Geometry check sheet. Reference: the model listing, model coordinates, mm. Give positions to 0.01 mm unless a question says otherwise; leave off trailing zeros. Write each loop counter-clockwise with the first axis right and the second up, starting at its lowest first coordinate (ties: lowest second). Pieces come first, ordered by that corner, then holes. Notation, with made-up numbers: M -14.5,28 L 3.5,28 A4 ccw 3.5,32 Z; hole C 89.5,51.25 d4. An arc over 180 degrees is marked long. Write each question's results on one line, items separated by ' | '.
```python
from build123d import *

# Parameters (mm, degrees)
SKETCH1_W            = 155
SKETCH1_H            = 103
SKETCH1_W_2          = 147
SKETCH1_H_2          = 95
BOSS_EXTRUDE2_DEPTH  = 3
SKETCH3_W            = 13
SKETCH3_H            = 3
BOSS_EXTRUDE5_DEPTH  = 22.5
SKETCH4_W            = 12
SKETCH4_H            = 3
BOSS_EXTRUDE6_DEPTH  = 22.5
SKETCH5_W            = 20
SKETCH5_H            = 32
SKETCH5_R            = 2.5
BOSS_EXTRUDE7_DEPTH  = 3
SKETCH6_W            = 20
SKETCH6_H            = 33
SKETCH6_R            = 2.5
BOSS_EXTRUDE8_DEPTH  = 3
SKETCH2_3_R          = 7
SKETCH2_3_R_2        = 1.25
BOSS_EXTRUDE11_DEPTH = 3
SKETCH2_R            = 7
SKETCH2_R_2          = 1.25
BOSS_EXTRUDE10_DEPTH = 3


with BuildPart() as part:
    # Sketch1 → Boss-Extrude2 (new body)
    with BuildSketch(Plane(origin=(0, 0, 0), x_dir=(1, 0, 0), z_dir=(0, 1, 0))):
        with Locations((77.5, 51.5)):
            Rectangle(SKETCH1_W, SKETCH1_H)
        with Locations((77.5, 51.5)):
            Rectangle(SKETCH1_W_2, SKETCH1_H_2, mode=Mode.SUBTRACT)
    extrude(amount=BOSS_EXTRUDE2_DEPTH)

    # Sketch3 → Boss-Extrude5 (add)
    with BuildSketch(Plane.ZY):
        with Locations((-51, 1.5)):
            Rectangle(SKETCH3_W, SKETCH3_H)
    extrude(amount=BOSS_EXTRUDE5_DEPTH)

    # Sketch4 → Boss-Extrude6 (add)
    with BuildSketch(Plane(origin=(155, 0, 0), x_dir=(0, 0, -1), z_dir=(1, 0, 0))):
        with Locations((51.5, 1.5)):
            Rectangle(SKETCH4_W, SKETCH4_H)
    extrude(amount=BOSS_EXTRUDE6_DEPTH)

    # Sketch5 → Boss-Extrude7 (add)
    with BuildSketch(Plane(origin=(0, 3, 0), x_dir=(1, 0, 0), z_dir=(0, 1, 0))):
        with Locations((187.5, 51.5)):
            Rectangle(SKETCH5_W, SKETCH5_H)
        with Locations(Location((187.5, 60.5, 0), (0, 0, 270))):
            Circle(SKETCH5_R, mode=Mode.SUBTRACT)
        with Locations(Location((187.5, 42.5, 0), (0, 0, 270))):
            Circle(SKETCH5_R, mode=Mode.SUBTRACT)
    extrude(amount=-BOSS_EXTRUDE7_DEPTH)

    # Sketch6 → Boss-Extrude8 (add)
    with BuildSketch(Plane(origin=(0, 3, 0), x_dir=(1, 0, 0), z_dir=(0, 1, 0))):
        with Locations((-32.378431073, 51.050390221)):
            Rectangle(SKETCH6_W, SKETCH6_H)
        with Locations(Location((-32.5, 60.5, 0), (0, 0, 270))):
            Circle(SKETCH6_R, mode=Mode.SUBTRACT)
        with Locations(Location((-32.5, 42.5, 0), (0, 0, 270))):
            Circle(SKETCH6_R, mode=Mode.SUBTRACT)
    extrude(amount=-BOSS_EXTRUDE8_DEPTH)

    # Sketch2_3 → Boss-Extrude11 (add)
    # profile 1 of 4: a face of its own
    with BuildSketch(Plane(origin=(0, 3, 0), x_dir=(1, 0, 0), z_dir=(0, 1, 0))):
        with Locations((8, 8)):
            Circle(SKETCH2_3_R)
        with Locations(Location((8, 8, 0), (0, 0, 270))):
            Circle(SKETCH2_3_R_2, mode=Mode.SUBTRACT)
    # profile 2 of 4: a face of its own
    with BuildSketch(Plane(origin=(0, 3, 0), x_dir=(1, 0, 0), z_dir=(0, 1, 0))):
        with Locations((146, 8.25)):
            Circle(SKETCH2_3_R)
        with Locations(Location((146, 8.25, 0), (0, 0, 270))):
            Circle(SKETCH2_3_R_2, mode=Mode.SUBTRACT)
    # profile 3 of 4: a face of its own
    with BuildSketch(Plane(origin=(0, 3, 0), x_dir=(1, 0, 0), z_dir=(0, 1, 0))):
        with Locations((8, 94.75)):
            Circle(SKETCH2_3_R)
        with Locations(Location((8, 94.75, 0), (0, 0, 270))):
            Circle(SKETCH2_3_R_2, mode=Mode.SUBTRACT)
    # profile 4 of 4: a face of its own
    with BuildSketch(Plane(origin=(0, 3, 0), x_dir=(1, 0, 0), z_dir=(0, 1, 0))):
        with Locations((146, 94.75)):
            Circle(SKETCH2_3_R)
        with Locations(Location((146, 94.75, 0), (0, 0, 270))):
            Circle(SKETCH2_3_R_2, mode=Mode.SUBTRACT)
    extrude(amount=-BOSS_EXTRUDE11_DEPTH)

    # Sketch2 → Boss-Extrude10 (add)
    # profile 1 of 4: a face of its own
    with BuildSketch(Plane(origin=(0, 3, 0), x_dir=(1, 0, 0), z_dir=(0, 1, 0))):
        with Locations((8, 8)):
            Circle(SKETCH2_R)
        with Locations(Location((8, 8, 0), (0, 0, 270))):
            Circle(SKETCH2_R_2, mode=Mode.SUBTRACT)
    # profile 2 of 4: a face of its own
    with BuildSketch(Plane(origin=(0, 3, 0), x_dir=(1, 0, 0), z_dir=(0, 1, 0))):
        with Locations((146, 8.25)):
            Circle(SKETCH2_R)
        with Locations(Location((146, 8.25, 0), (0, 0, 270))):
            Circle(SKETCH2_R_2, mode=Mode.SUBTRACT)
    # profile 3 of 4: a face of its own
    with BuildSketch(Plane(origin=(0, 3, 0), x_dir=(1, 0, 0), z_dir=(0, 1, 0))):
        with Locations((8, 94.75)):
            Circle(SKETCH2_R)
        with Locations(Location((8, 94.75, 0), (0, 0, 270))):
            Circle(SKETCH2_R_2, mode=Mode.SUBTRACT)
    # profile 4 of 4: a face of its own
    with BuildSketch(Plane(origin=(0, 3, 0), x_dir=(1, 0, 0), z_dir=(0, 1, 0))):
        with Locations((146, 94.75)):
            Circle(SKETCH2_R)
        with Locations(Location((146, 94.75, 0), (0, 0, 270))):
            Circle(SKETCH2_R_2, mode=Mode.SUBTRACT)
    extrude(amount=-BOSS_EXTRUDE10_DEPTH)


solid = part.part
```
Q1. Release check for a two-part mould opening along X. For faces 1 (the face through (13, 1.5, -12.9)), 2 (the face through (77, 3, -101)) record: released by +X, released by -X, zero draft, split by the parting line, or undercut.
Answer key:
face 1: undercut | face 2: zero draft
Q2. Section check B-B (z = -23). Enter the section's corners in (x, y), then the cut area to 3 significant figures.
Answer key:
outline: M 0,0 L 4,0 L 4,3 L 0,3 Z; M 151,0 L 155,0 L 155,3 L 151,3 Z | area: 24.0 mm2
Q3. Section check D-D (y = 1.2). State how many separate pieces and enclosed holes the cut face has, then the cut area to 3 significant figures.
Answer key:
separate pieces: 1 | enclosed holes: 9 | area: 4,220 mm2
Q4. Material ranges on probe 1 along X at (y, z) = (1.35, -8.25); probe 2 along X at (y, z) = (2.7, -31); probe 3 along Z at (x, y) = (80, 2.45), recorded low to high. Write a range as [from, to].
Answer key:
probe 1: x = [0, 6.78], [9.22, 15], [139, 144.75], [147.25, 155] | probe 2: x = [0, 4], [151, 155] | probe 3: z = [-103, -99], [-4, 0]
Q5. Section check C-C (z = -60.5). Enter the section's corners in (x, y), then the cut area to 3 significant figures.
Answer key:
outline: M -42.38,0 L -35,0 L -35,3 L -42.38,3 Z; M -30,0 L -22.38,0 L -22.38,3 L -30,3 Z; M 0,0 L 4,0 L 4,3 L 0,3 Z; M 151,0 L 155,0 L 155,3 L 151,3 Z; M 177.5,0 L 185,0 L 185,3 L 177.5,3 Z; M 190,0 L 197.5,0 L 197.5,3 L 190,3 Z | area: 114 mm2
Q6. Depth check by flat-ended pin: P1, Ø1.5, axis at x = 162, y = 1.5, coming from the -Z side; P2, Ø1.5, axis at y = 1.5, z = -90.5, coming from the +X side; P3, Ø1.5, axis at x = 188.5, y = 2, coming from the +Z side. Enter the tip coordinate at first touch or a pass-through.
Answer key:
P1: stops at z = -57.5 | P2: stops at x = 155 | P3: stops at z = -35.5
Q7. Section check A-A (x = 121). Enter the section's corners in (y, z).
Answer key:
outline: M 0,-103 L 3,-103 L 3,-99 L 0,-99 Z; M 0,-4 L 3,-4 L 3,0 L 0,0 Z
